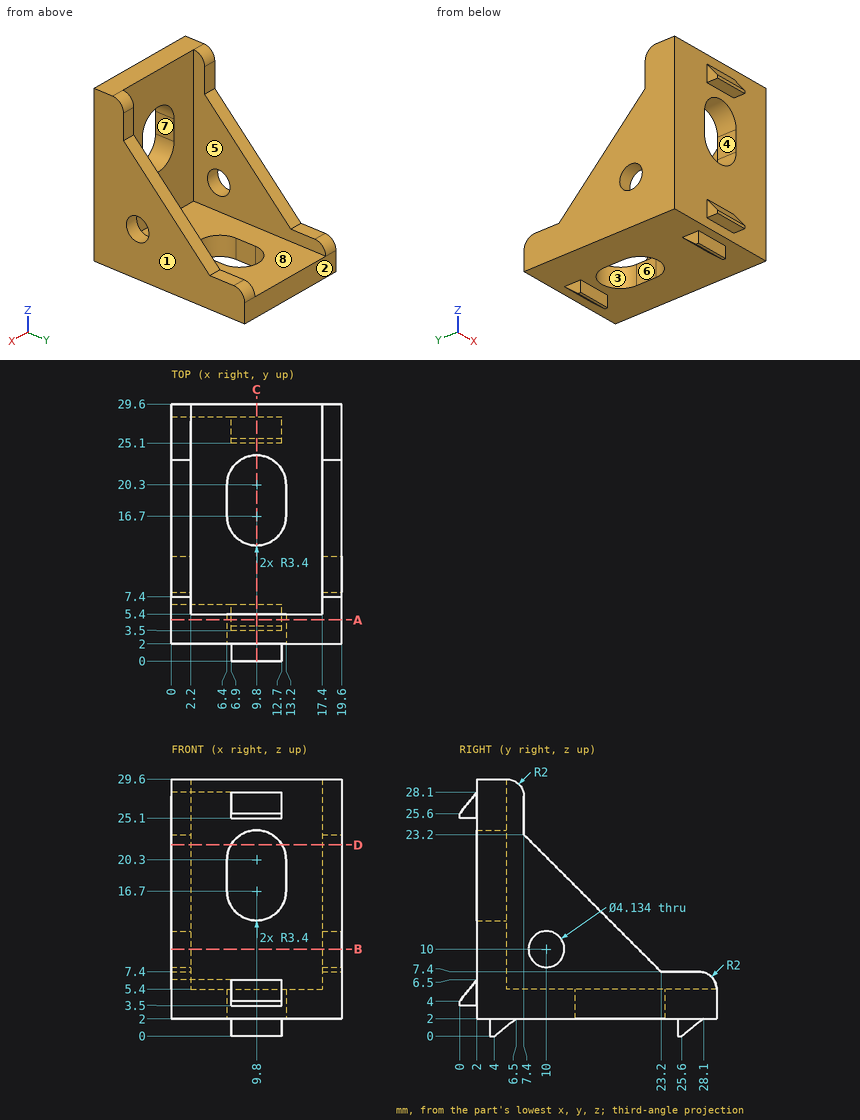
Part print with two shaded views. Sizes in mm from the minimum x, y, z corner. A direction names the side the tool comes from. Give positions to 0.01 mm unless a question says otherwise; leave off trailing zeros. Order: outer loops, then holes, each group sorted by start corner. A loop starts at its lowest first (then second) coordinate and runs counter-clockwise, first axis right, second up.
1) 3-axis set-ups, long thin cutter, end or side, ignore diameter. For the marked faces 1, 2, 3, 4 and 5: which of +Z, -Z, +X, -X, +Y, -Y reach the whole face in a straight line?
2) Saw through at A-A, the plane y = 4.75. Write the cut outline in (x, z), then the cut area to 3 significant figures.
3) Wall check: probe 1 along X at (y, z) = (10.5, 12.75); probe 2 along Z at (x, y) = (14.5, 21). Give the ranges that are in metal, low to high.
4) Saw through at B-B, the plane z = 10. Write the cut outline in (x, y), then the cut area to 3 significant figures.
5) Pin check, flat tips, straight feed: pin 1 (0.6 mm diameter, centred on x = 11, y = 1, fed in from -Z); pin 2 (1.5 mm diameter, centred on x = 4, z = 8, fed in from +Y); pin 3 (1.8 mm diameter, centred on x = 19, y = 24.5, fed in from +Z); pin 4 (1.5 mm diameter, centred on y = 26, z = 10, fed in from -X). Stop position of each tip, or through.
6) Saw through at C-C, the plane x = 9.8. Count the separate pieces of the cut face and the enclosed holes in it, then the cut area to 3 significant figures.
7) Saw through at D-D, the plane z = 22. Write the cut outline in (x, y).
8) Mould opens along Z. For the marked faces 6, 7 and 8 say: +Z half, -Z half, draft (parallel to the pull), parting line (faces both ways), or undercut.
Computed:
1. face 1: +Z, -Z, +X, +Y, -Y
1. face 2: +Z, -Z, +X, -X, +Y
1. face 3: +Z, -Z
1. face 4: +Y, -Y
1. face 5: +Z, +Y
2. outline: (0, 2) - (6.9, 2) - (6.9, 0.6) - (12.7, 0.6) - (12.7, 2) - (19.6, 2) - (19.6, 29.6) - (0, 29.6) - close; hole (6.4, 16.7) arc R3.4 ccw to (13.2, 16.7) - (13.2, 20.3) arc R3.4 ccw to (6.4, 20.3) - close
2. area: 488 mm2
3. probe 1: x = 0 to 2.2, 17.4 to 19.6
3. probe 2: z = 2 to 5.4
4. outline: (0, 2) - (19.6, 2) - (19.6, 7.93) - (17.4, 7.93) - (17.4, 5.4) - (2.2, 5.4) - (2.2, 7.93) - (0, 7.93) - close; (0, 12.07) - (2.2, 12.07) - (2.2, 20.6) - (0, 20.6) - close; (17.4, 12.07) - (19.6, 12.07) - (19.6, 20.6) - (17.4, 20.6) - close
4. area: 115 mm2
5. pin 1: stops at z = 3.5
5. pin 2: stops at y = 5.4
5. pin 3: stops at z = 7.4
5. pin 4: passes through
6. separate pieces: 3
6. enclosed holes: 0
6. area: 119 mm2
7. outline: (0, 2) - (6.86, 2) - (6.86, 5.4) - (2.2, 5.4) - (2.2, 8.6) - (0, 8.6) - close; (12.74, 2) - (19.6, 2) - (19.6, 8.6) - (17.4, 8.6) - (17.4, 5.4) - (12.74, 5.4) - close
8. face 6: draft
8. face 7: undercut
8. face 8: +Z half
